Can you work these out from the model? Positions are in its coordinate system, mm. Coordinates: 2 decimals unless noted, no trailing zeros. Order: outer loops, then holes, each group sorted by start corner. A loop starts at its lowest first (then second) coordinate and runs counter-clockwise, first axis right, second up. Notation, with made-up numbers: (10, -22.75) -> (34, -22.75) arc R19 cw to (34, -2.75) -> close; hole circle Ø6 at (-28, 9.25). An arc over 180 degrees is marked (long way). Answer as a JSON object with one key per item and string values. Group by question number.
(1) I need wall thicknesses on line 1 (X direction, y = 5.5, z = -38); line 2 (X direction, y = 5, z = 7.5); line 3 (Z direction, x = 136, y = 4.5). Which ranges of each line are inside material? Lowest first, please.
(2) If we mould it in two halves opening along X, with no side actions, what happens to faces 1 (the cylindrical face through (-82.539, 3.131, -75.773)), 2 (the flat face through (0, 3, -165.422)), 3 (the flat face through (152.349, 3, -52))? For each: pulls with the +X half, pulls with the -X half, needs draft (parallel to the pull), parting line crosses it, or undercut.
(3) I want a section at A-A, the plane y = 3.5. State how many separate pieces and enclosed holes the cut face has, plus the area to 3 significant figures.
(4) I want a section at B-B, the plane x = 67.5. List the corners of the cut face in (y, z) for me, plus the area to 3 significant figures.
from build123d import *

# Parameters (mm, degrees)
SKETCH1_R           = 4.85
SKETCH1_R_2         = 2.5
SKETCH1_R_3         = 17.5
BOSS_EXTRUDE1_DEPTH = 6.35
SKETCH5_R           = 2
CUT_EXTRUDE2_DEPTH  = 10


with BuildPart() as part:
    # Sketch1 → Boss-Extrude1 (new body)
    with BuildSketch(Plane(origin=(0, 0, 0), x_dir=(1, 0, 0), z_dir=(0, 1, 0))):
        with BuildLine():
            Line((-132.651439051, 165.421561199), (137.348560949, 165.421561199))
            ThreePointArc((137.348560949, 165.421561199), (147.955162667, 161.028162917), (152.348560949, 150.421561199))
            Line((152.348560949, 150.421561199), (152.348560949, -49.578438801))
            ThreePointArc((152.348560949, -49.578438801), (147.955162667, -60.185040519), (137.348560949, -64.578438801))
            Line((137.348560949, -64.578438801), (-132.651439051, -64.578438801))
            ThreePointArc((-132.651439051, -64.578438801), (-143.258040769, -60.185040519), (-147.651439051, -49.578438801))
            Line((-147.651439051, -49.578438801), (-147.651439051, 150.421561199))
            ThreePointArc((-147.651439051, 150.421561199), (-143.258040769, 161.028162917), (-132.651439051, 165.421561199))
        make_face()
        with Locations((-132.651439051, 150.421561199)):
            Circle(SKETCH1_R, mode=Mode.SUBTRACT)
        with Locations((137.348560949, -49.578438801)):
            Circle(SKETCH1_R, mode=Mode.SUBTRACT)
        with Locations((-45.081439051, 109.991561199)):
            Circle(SKETCH1_R_2, mode=Mode.SUBTRACT)
        with Locations((-45.081439051, 62.851561199)):
            Circle(SKETCH1_R_2, mode=Mode.SUBTRACT)
        with Locations((-92.221439051, 62.851561199)):
            Circle(SKETCH1_R_2, mode=Mode.SUBTRACT)
        with Locations((-92.221439051, 109.991561199)):
            Circle(SKETCH1_R_2, mode=Mode.SUBTRACT)
        with Locations((49.778560949, 37.991561199)):
            Circle(SKETCH1_R_2, mode=Mode.SUBTRACT)
        with Locations((96.918560949, 37.991561199)):
            Circle(SKETCH1_R_2, mode=Mode.SUBTRACT)
        with Locations((96.918560949, -9.148438801)):
            Circle(SKETCH1_R_2, mode=Mode.SUBTRACT)
        with Locations((49.778560949, -9.148438801)):
            Circle(SKETCH1_R_2, mode=Mode.SUBTRACT)
        with Locations((137.348560949, 150.421561199)):
            Circle(SKETCH1_R, mode=Mode.SUBTRACT)
        with Locations((-132.651439051, -49.578438801)):
            Circle(SKETCH1_R, mode=Mode.SUBTRACT)
        with Locations((-68.651439051, 86.421561199)):
            Circle(SKETCH1_R_3, mode=Mode.SUBTRACT)
        with Locations((73.348560949, 14.421561199)):
            Circle(SKETCH1_R_3, mode=Mode.SUBTRACT)
    extrude(amount=BOSS_EXTRUDE1_DEPTH)

    # Sketch5 → Cut-Extrude2 (cut)
    with BuildSketch(Plane.XZ):
        with Locations((-97.651439051, -5.421561199)):
            Circle(SKETCH5_R)
        with Locations((11.348560949, -5.421561199)):
            Circle(SKETCH5_R)
        with Locations((-6.651439051, -95.421561199)):
            Circle(SKETCH5_R)
        with Locations((102.348560949, -95.421561199)):
            Circle(SKETCH5_R)
    extrude(amount=-CUT_EXTRUDE2_DEPTH, mode=Mode.SUBTRACT)


solid = part.part
Computed values:
{
 "1": {"line 1": "x = -147.65 to 47.28, 52.28 to 94.42, 99.42 to 152.35", "line 2": "x = -147.65 to 47.9, 51.66 to 95.04, 98.8 to 152.35", "line 3": "z = -165.42 to -155.08, -145.76 to 44.92, 54.24 to 64.58"},
 "2": {"face 1": "undercut", "face 2": "needs draft", "face 3": "pulls with the +X half"},
 "3": {"separate pieces": "1", "enclosed holes": "18", "area": "66,400 mm2"},
 "4": {"outline": "(0, -165.42) -> (6.35, -165.42) -> (6.35, -30.92) -> (0, -30.92) -> close; (0, 2.07) -> (6.35, 2.07) -> (6.35, 64.58) -> (0, 64.58) -> close", "area": "1,250 mm2"}
}
